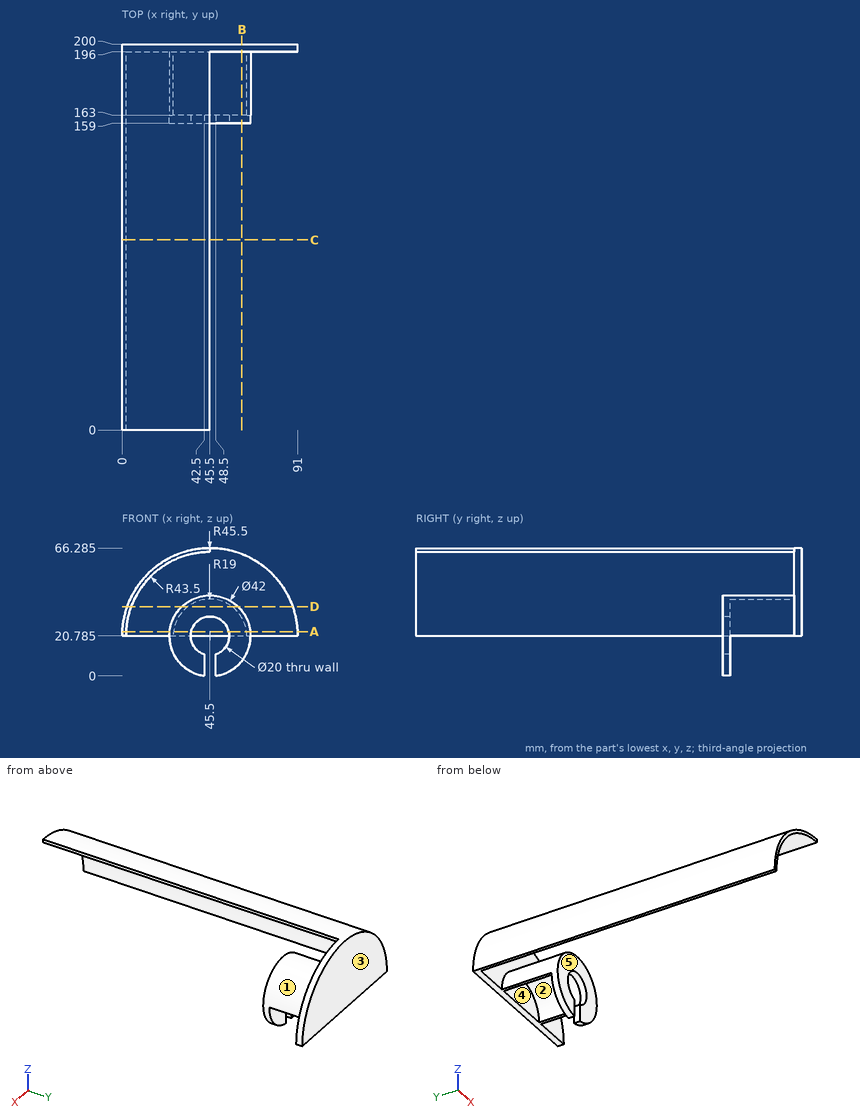
Print and shaded views of the part. All mm, measured from the part's lowest x, y and z. A direction names the side the tool comes from. Coordinates: 2 decimals unless noted, no trailing zeros. Order: outer loops, then holes, each group sorted by start corner. A loop starts at its lowest first (then second) coordinate and runs counter-clockwise, first axis right, second up.
Item 1: Tool access for the marked faces 1 and 2: list every direction of +Z, -Z, +X, -X, +Y, -Y with a clear straight run to the whole face (end or side of a thin tool).
Filled in:
face 1: -Y
face 2: -Z
Item 2: Drill centre lines: L1, parallel to Z at x = 45, y = 161; L2, parallel to Y at x = 57, z = 34; L3, parallel to Y at x = 87, z = 34.5. Where is each one in solid material? Low to high.
Filled in:
L1: z = 30.77 to 41.78, 64.28 to 66.28
L2: y = 159 to 163, 196 to 200
L3: y = 196 to 200
Item 3: Saw through at D-D on z = 36. List the corners of the cut face in (x, y), then the cut area to 3 significant figures.
Filled in:
outline: (2.62, 0) - (4.75, 0) - (4.75, 196) - (31.03, 196) - (31.03, 159) - (59.97, 159) - (59.97, 196) - (88.38, 196) - (88.38, 200) - (2.62, 200) - close; hole (34.12, 163) - (56.88, 163) - (56.88, 196) - (34.12, 196) - close
area: 1,080 mm2
Item 4: Saw through at C-C on y = 98.5. List the corners of the cut face in (x, z) (1 decimal), then the cut area to 3 significant figures.
Filled in:
outline: (0, 20.8) - (2, 20.8) arc R43.5 cw to (45.5, 64.3) - (45.5, 66.3) arc R45.5 ccw to start
area: 140 mm2
Item 5: Saw through at B-B on x = 62. List the corners of the cut face in (y, z) (1 decimal), then the cut area to 3 significant figures.
Filled in:
outline: (159, 7.8) - (163, 7.8) - (163, 30.2) - (196, 30.2) - (196, 20.8) - (200, 20.8) - (200, 63.2) - (196, 63.2) - (196, 33.8) - (159, 33.8) - close
area: 391 mm2
Item 6: Drop flat-ended pins along their axis: pin 1 Ø10 at (x, y) = (71, 168) entering from -Z (1 decimal); pin 2 Ø16 at (x, z) = (45.5, 20.78) entering from -Y; pin 3 Ø5.5 at (x, z) = (44, 31.5) entering from -Y. Give the stop position or say it passes through.
Filled in:
pin 1: stops at z = 20.8
pin 2: stops at y = 196
pin 3: stops at y = 159
Item 7: Saw through at A-A on z = 23. List the corners of the cut face in (x, y).
Filled in:
outline: (0.05, 0) - (2.06, 0) - (2.06, 196) - (24.62, 196) - (24.62, 159) - (35.75, 159) - (35.75, 163) - (26.63, 163) - (26.63, 196) - (64.37, 196) - (64.37, 163) - (55.25, 163) - (55.25, 159) - (66.38, 159) - (66.38, 196) - (90.95, 196) - (90.95, 200) - (0.05, 200) - close
Item 8: Mould opens along Y. For the marked faces 3, 4 and 5 say: released by +Y, released by -Y, zero draft, split by the parting line, or undercut.
Filled in:
face 3: released by +Y
face 4: undercut
face 5: released by -Y
